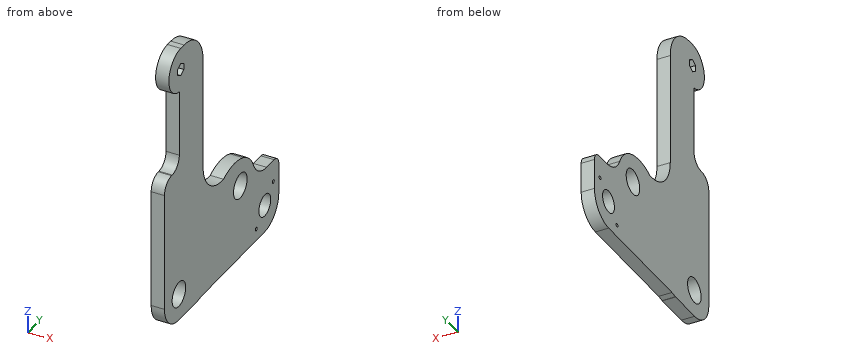
```python
from build123d import *

# Parameters (mm, degrees)
SALIENTE_EXTRUIR1_DEPTH = 15
CORTAR_EXTRUIR1_DEPTH   = 477.91260816
REDONDEO1_R             = 220
REDONDEO2_R             = 70
REDONDEO3_R             = 15
REDONDEO4_R             = 30
CROQUIS7_R              = 14.29
CORTAR_EXTRUIR5_DEPTH   = 477.91260816
CROQUIS8_R              = 14.29
CORTAR_EXTRUIR6_DEPTH   = 523
CORTAR_EXTRUIR12_DEPTH  = 477.91260816
REDONDEO5_R             = 40
CORTAR_EXTRUIR13_DEPTH  = 429.85874997
REDONDEO6_R             = 40
SALIENTE_EXTRUIR3_DEPTH = 15
SALIENTE_EXTRUIR4_DEPTH = 15
CROQUIS21_R             = 2.02
CROQUIS21_R_2           = 12.5
CORTAR_EXTRUIR17_DEPTH  = 450.880285455
REDONDEO7_R             = 30


with BuildPart() as part:
    # Croquis1 → Saliente-Extruir1 (new body)
    with BuildSketch(Plane(origin=(0, 0, 0), x_dir=(0, 0, -1), z_dir=(1, 0, 0))):
        with BuildLine():
            Line((65, 25.4), (65, 281.06162282))
            Line((65, 281.06162282), (385, 281.06162282))
            Line((385, 281.06162282), (385, -8.93837718))
            Line((385, -8.93837718), (205, -8.93837718))
            Line((205, -8.93837718), (205, 22.4))
            Line((205, 22.4), (115, 22.4))
            Line((115, 22.4), (114.819347292, 22.4))
            ThreePointArc((114.819347292, 22.4), (88.497282844, 0.445204045), (65, 25.4))
        make_face()
    extrude(amount=SALIENTE_EXTRUIR1_DEPTH)

    # Croquis2 → Cortar-Extruir1 (cut, through all)
    with BuildSketch(Plane.ZY):
        Polygon((-82.667651581, 25.4), (-86.333825791, 31.75), (-93.666174209, 31.75), (-97.332348419, 25.4), (-93.666174209, 19.05), (-86.333825791, 19.05), align=None)
    extrude(amount=-CORTAR_EXTRUIR1_DEPTH, mode=Mode.SUBTRACT)

    # Redondeo1
    redondeo1_edges = [part.edges().sort_by_distance(p)[0] for p in [
        (7.5, 281.06162282, -385),
    ]]
    fillet(redondeo1_edges, radius=REDONDEO1_R)

    # Redondeo2
    redondeo2_edges = [part.edges().sort_by_distance(p)[0] for p in [
        (7.5, 281.06162282, -65),
    ]]
    fillet(redondeo2_edges, radius=REDONDEO2_R)

    # Redondeo3
    redondeo3_edges = [part.edges().sort_by_distance(p)[0] for p in [
        (7.5, -8.93837718, -205),
        (7.5, 22.4, -205),
    ]]
    fillet(redondeo3_edges, radius=REDONDEO3_R)

    # Redondeo4
    redondeo4_edges = [part.edges().sort_by_distance(p)[0] for p in [
        (7.5, -8.93837718, -385),
    ]]
    fillet(redondeo4_edges, radius=REDONDEO4_R)

    # Croquis7 → Cortar-Extruir5 (cut, through all)
    with BuildSketch(Plane(origin=(15, 0, 0), x_dir=(0, 0, -1), z_dir=(1, 0, 0))):
        with Locations((354.499999998, 21.561622823)):
            Circle(CROQUIS7_R)
    extrude(amount=-CORTAR_EXTRUIR5_DEPTH, mode=Mode.SUBTRACT)

    # Croquis8 → Cortar-Extruir6 (cut)
    with BuildSketch(Plane(origin=(15, 0, 0), x_dir=(0, 0, -1), z_dir=(1, 0, 0))):
        with Locations((299.999999998, 151.061622823)):
            Circle(CROQUIS8_R)
    extrude(amount=-CORTAR_EXTRUIR6_DEPTH, mode=Mode.SUBTRACT)

    # Croquis14 → Cortar-Extruir12 (cut, through all)
    with BuildSketch(Plane(origin=(15, 0, 0), x_dir=(0, 0, -1), z_dir=(1, 0, 0))):
        with BuildLine():
            Line((65, 72.4), (270, 72.4))
            ThreePointArc((270, 72.4), (274.363902477, 93.8541681), (271.886825139, 115.607077367))
            ThreePointArc((271.886825139, 115.607077367), (293.695729554, 182.870527237), (360.959179423, 161.06162282))
            Line((360.959179423, 161.06162282), (409.037931036, 257.33581614))
            Line((409.037931036, 257.33581614), (105.335360325, 302.08857435))
            Line((105.335360325, 302.08857435), (0, 212.58305793))
            Line((0, 212.58305793), (65, 72.4))
        make_face()
    extrude(amount=-CORTAR_EXTRUIR12_DEPTH, mode=Mode.SUBTRACT)

    # Redondeo5
    # the kernel refuses this fillet: 40 mm, written as the material it adds along each edge
    with BuildSketch(Plane(origin=(15, 72.4, -270), x_dir=(0, 0.9990478553762716, -0.0436277740444352), z_dir=(-1, 0, 0))) as redondeo5_piece_1:
        with BuildLine():
            CenterArc((38.304739361, -39.69334508), REDONDEO5_R, 82.900783034, 94.598735986)
            Line((-1.657174854, -37.948234118), (0, 0))
            ThreePointArc((0, 0), (21.624127981, 3.423749812), (43.248255961, 0))
        make_face()
    extrude(amount=15)
    # the kernel refuses this fillet: 40 mm, written as the material it takes off along each edge
    with BuildSketch(Plane(origin=(115, 72.4, -65), x_dir=(0, 0, -1), z_dir=(-1, 0, 0))) as redondeo5_2_piece_1:
        with BuildLine():
            CenterArc((REDONDEO5_R, REDONDEO5_R), REDONDEO5_R, 180, 90)
            Line((0, REDONDEO5_R), (0, 0))
            Line((0, 0), (REDONDEO5_R, 0))
        make_face()
    extrude(amount=215, mode=Mode.SUBTRACT)

    # Croquis15 → Cortar-Extruir13 (cut, through all)
    with BuildSketch(Plane(origin=(15, 0, 0), x_dir=(0, 0, -1), z_dir=(1, 0, 0))):
        with BuildLine():
            Line((316.423002092, 188.334350095), (358.626196651, 190.922485323))
            Line((358.626196651, 190.922485323), (422.761195779, 101.20409943))
            Line((422.761195779, 101.20409943), (385, 21.06162282))
            ThreePointArc((385, 21.06162282), (371.881027209, 113.376882145), (316.423002092, 188.334350095))
        make_face()
    extrude(amount=-CORTAR_EXTRUIR13_DEPTH, mode=Mode.SUBTRACT)

    # Redondeo6
    # the kernel refuses this fillet: 40 mm, written as the material it takes off along each edge
    with BuildSketch(Plane(origin=(154.505258901, 188.334350095, -316.423002092), x_dir=(0, -0.5580210387188341, 0.8298268014153035), z_dir=(-1, 0, 0))) as redondeo6_piece_1:
        with BuildLine():
            CenterArc((33.481262136, -33.19307214), REDONDEO6_R, 56.080950646, 115.615192876)
            ThreePointArc((-6.099380682, -27.416159984), (-3.556977801, -13.59522176), (0, 0))
            ThreePointArc((0, 0), (27.90105178, 8.508659825), (55.802103561, 0))
        make_face()
    extrude(amount=294.010517803, mode=Mode.SUBTRACT)

    # Croquis18 → Saliente-Extruir3 (add, through all)
    with BuildSketch(Plane.ZY):
        with BuildLine():
            Line((-336.783225667, 168.987268689), (-324.9259333, 170.954067241))
            Line((-324.9259333, 170.954067241), (-309.780230989, 182.020805528))
            ThreePointArc((-309.780230989, 182.020805528), (-329.588467491, 188.570394011), (-336.783225667, 168.987268689))
        make_face()
    extrude(amount=-SALIENTE_EXTRUIR3_DEPTH)

    # Croquis20 → Saliente-Extruir4 (add, through all)
    with BuildSketch(Plane.ZY):
        with BuildLine():
            Line((-384.080413654, 202.254755045), (-384.080413654, 68.806205343))
            Line((-384.080413654, 68.806205343), (-355.955719628, 128.198236155))
            Line((-355.955719628, 128.198236155), (-350.988918253, 138.686827429))
            Line((-350.988918253, 138.686827429), (-333.391481861, 167.902196457))
            Line((-333.391481861, 167.902196457), (-333.391481861, 179.145496263))
            Line((-333.391481861, 179.145496263), (-331.848601066, 185.40903393))
            Line((-331.848601066, 185.40903393), (-327.722665886, 187.904048047))
            Line((-327.722665886, 187.904048047), (-321.465563641, 187.904048047))
            Line((-321.465563641, 187.904048047), (-315.23558207, 184.151512718))
            Line((-315.23558207, 184.151512718), (-309.780230989, 182.020805528))
            Line((-309.780230989, 182.020805528), (-309.780230989, 222.254755045))
            ThreePointArc((-309.780230989, 222.254755045), (-312.709163177, 229.325822857), (-319.780230989, 232.254755045))
            Line((-319.780230989, 232.254755045), (-354.080413654, 232.254755045))
            ThreePointArc((-354.080413654, 232.254755045), (-375.293617089, 223.467958481), (-384.080413654, 202.254755045))
        make_face()
    extrude(amount=-SALIENTE_EXTRUIR4_DEPTH)

    # Croquis21 → Cortar-Extruir17 (cut, through all)
    with BuildSketch(Plane.ZY):
        with Locations((-334.74499674, 220.62921413)):
            Circle(CROQUIS21_R)
        with Locations((-370.666021225, 184.708189645)):
            Circle(CROQUIS21_R)
        with Locations((-352.705508983, 202.668701887)):
            Circle(CROQUIS21_R_2)
    extrude(amount=-CORTAR_EXTRUIR17_DEPTH, mode=Mode.SUBTRACT)

    # Redondeo7
    redondeo7_edges = [part.edges().sort_by_distance(p)[0] for p in [
        (7.5, 182.020805528, -309.780230989),
    ]]
    fillet(redondeo7_edges, radius=REDONDEO7_R)


solid = part.part
```
Work out the finished part from the listing and answer in its coordinate system (mm). Give positions to 0.01 mm unless a question says otherwise; leave off trailing zeros. Loops run counter-clockwise (first coordinate to the right, second up) from the corner with the lowest first, then second, coordinate; pieces in that order, holes last. Notation, with made-up numbers: M -9,82.5 L 24,82.5 A36 cw 24,119.5 Z; hole C 21.25,65.25 d11. An arc over 180 degrees is marked long. One line per item, written item: value. Start each with the question number.
1. Find the intervals of material crossed by probe 1 along Y at (x, z) = (8.5, -354.5); probe 2 along Y at (x, z) = (1.25, -229); probe 3 along Z at (x, y) = (14, 140), in increasing order.
2. Find section B-B (x = 8). State how many separate pieces and enclosed holes the cut face has, and give its area (3 significant figures).
3. Each of these flat-tipped pins is pushed along its axis until it touches: P1, Ø3.5, axis at x = 10.5, z = -91.5, coming from the +Y side; P2, Ø7.5, axis at x = 9.5, z = -175, coming from the +Y side; P3, Ø2, axis at x = 10.5, z = -89, coming from the -Y side. Where does it stop, or does it pass through?
4. Find section C-C (z = -360.5). Give the vertices of the cut face in (x, y).
5. Find section A-A (z = -90). Give the vertices of the cut face in (x, y).
6. Find section D-D (y = 125). Give the vertices of the cut face in (x, z).
Reported:
1. probe 1: y = -8.94 to 7.27, 35.85 to 190.3, 215.04 to 232.25
1. probe 2: y = -8.94 to 72.4
1. probe 3: z = -384.08 to -309.05, -290.95 to -266.45
2. separate pieces: 1
2. enclosed holes: 6
2. area: 36,200 mm²
3. P1: stops at y = 70.64
3. P2: stops at y = 72.4
3. P3: stops at y = 0.4
4. outline: M 0,-8.43 L 15,-8.43 L 15,8.59 L 0,8.59 Z; M 0,34.53 L 15,34.53 L 15,192.9 L 0,192.9 Z; M 0,212.44 L 15,212.44 L 15,231.56 L 0,231.56 Z
5. outline: M 0,0.4 L 15,0.4 L 15,19.05 L 0,19.05 Z; M 0,31.75 L 15,31.75 L 15,69.48 L 0,69.48 Z
6. outline: M 0,-384.08 L 15,-384.08 L 15,-268.23 L 0,-268.23 Z
